from build123d import *

# Parameters (mm, degrees)
BOSS_EXTRUDE3_DEPTH = 6


with BuildPart() as part:
    # Sketch1 → Boss-Extrude3 (new body)
    with BuildSketch(Plane(origin=(0, 0, 0), x_dir=(1, 0, 0), z_dir=(0, 1, 0))):
        with BuildLine():
            ThreePointArc((-76.2, 131.982271537), (-131.982271537, 76.2), (-152.4, 0))
            Line((-152.4, 0), (-609.6, 0))
            ThreePointArc((-609.6, 0), (-527.929086147, 304.8), (-304.8, 527.929086147))
            Line((-304.8, 527.929086147), (-76.2, 131.982271537))
        make_face()
        with BuildLine():
            Line((-335.2, 10), (-599.516605275, 10))
            ThreePointArc((-599.516605275, 10), (-578.516992176, 157.601553812), (-521.750777563, 295.459449184))
            Line((-521.750777563, 295.459449184), (-335.2, 187.75430754))
            Line((-335.2, 187.75430754), (-335.2, 10))
        make_face(mode=Mode.SUBTRACT)
        with BuildLine():
            Line((-89.706166951, 135.375638912), (-171.260254038, 276.631461311))
            Line((-171.260254038, 276.631461311), (-325.2, 187.75430754))
            Line((-325.2, 187.75430754), (-325.2, 10))
            Line((-325.2, 10), (-162.091825827, 10))
            ThreePointArc((-162.091825827, 10), (-140.642525575, 81.2), (-89.706166951, 135.375638912))
        make_face(mode=Mode.SUBTRACT)
        with BuildLine():
            Line((-330.2, 196.414561578), (-516.750777563, 304.119703222))
            ThreePointArc((-516.750777563, 304.119703222), (-425.745445365, 422.209634839), (-308.418556675, 514.196610158))
            Line((-308.418556675, 514.196610158), (-176.260254038, 285.291715349))
            Line((-176.260254038, 285.291715349), (-330.2, 196.414561578))
        make_face(mode=Mode.SUBTRACT)
    extrude(amount=BOSS_EXTRUDE3_DEPTH)


solid = part.part
Could you check a few things on this model? Use its own coordinates, in mm. A direction names the side the tool comes from. Round coordinates to 2 decimals unless told otherwise and drop trailing zeros. Order: outer loops, then holes, each group sorted by start corner. A loop starts at its lowest first (then second) coordinate and runs counter-clockwise, first axis right, second up.
Q1. Imagine slicing it at A-A, the plane y = 3.6. List the corners of the cut face in (x, z) for me, then the cut area to 3 significant figures.
Geometry says:
outline: (-609.6, 0) arc R609.6 ccw to (-304.8, -527.93) - (-76.2, -131.98) arc R152.4 cw to (-152.4, 0) - close; hole (-599.52, -10) arc R599.6 ccw to (-521.75, -295.46) - (-335.2, -187.75) - (-335.2, -10) - close; hole (-516.75, -304.12) arc R599.6 ccw to (-308.42, -514.2) - (-176.26, -285.29) - (-330.2, -196.41) - close; hole (-325.2, -187.75) - (-171.26, -276.63) - (-89.71, -135.38) arc R162.4 cw to (-162.09, -10) - (-325.2, -10) - close
area: 22,500 mm2
Q2. Which directions (+Z, -Z, +X, -X, +Y, -Y) give clear straight access to the entire face, cutting with the end or side of a thin tool? Please do faces 4 (the face through (-427.22, 2.96, -420.72)), 5 (the face through (-361, 0, -207)).
Geometry says:
face 4: +Y, -Y
face 5: +Z, -Z, +X, -X, -Y
Q3. I'm going to push flat-ended pins straight in: P1, Ø1.8, axis at y = 2.5, z = -132, coming from the +X side; P2, Ø3, axis at x = -223, y = 1.5, coming from the -Z side; P3, Ø1.5, axis at x = -524.5, y = 5.5, coming from the -Z side; P4, Ø1.5, axis at x = -177.5, z = -285, coming from the -Y side. Where does each tip first touch, or does it pass through?
Geometry says:
P1: stops at x = -76.2
P2: stops at z = -388.85
P3: stops at z = -311.93
P4: stops at y = 0
Q4. Imagine slicing it at B-B, the plane x = -384. List the corners of the cut face in (y, z) for me, then the cut area to 3 significant figures.
Geometry says:
outline: (0, -473.45) - (6, -473.45) - (6, -460.5) - (0, -460.5) - close; (0, -227.48) - (6, -227.48) - (6, -215.93) - (0, -215.93) - close; (0, -10) - (6, -10) - (6, 0) - (0, 0) - close
area: 207 mm2
Q5. Imagine slicing it at C-C, the plane z = -230.5. List the corners of the cut face in (x, y) for me.
Geometry says:
outline: (-564.34, 0) - (-553.52, 0) - (-553.52, 6) - (-564.34, 6) - close; (-409.24, 0) - (-389.24, 0) - (-389.24, 6) - (-409.24, 6) - close; (-271.16, 0) - (-251.16, 0) - (-251.16, 6) - (-271.16, 6) - close; (-144.63, 0) - (-133.08, 0) - (-133.08, 6) - (-144.63, 6) - close
Q6. Imagine slicing it at D-D, the plane z = -433.5. List the corners of the cut face in (x, y) for me.
Geometry says:
outline: (-428.59, 0) - (-414.24, 0) - (-414.24, 6) - (-428.59, 6) - close; (-261.83, 0) - (-250.28, 0) - (-250.28, 6) - (-261.83, 6) - close
Q7. Thinking about a two-plate mould opening in X: for faces 1 (the face through (-247.153, 2.958, -232.815)), 2 (the face through (-131.4, 3, -77.2)), 3 (the face through (-361, 6, -207)), which applies, released by +X, released by -X, zero draft, split by the parting line, or undercut?
Geometry says:
face 1: undercut
face 2: released by +X
face 3: zero draft
Q8. Please list where these lines run through material, in increasing order: probe 1 along Z at (x, y) = (-471, 0.5); probe 2 along X at (y, z) = (1.9, -69.5); probe 3 along Z at (x, y) = (-463.5, 2.1).
Geometry says:
probe 1: z = -387 to -371.05, -277.71 to -266.16, -10 to 0
probe 2: x = -605.63 to -595.56, -335.2 to -325.2, -146.78 to -135.63
probe 3: z = -395.95 to -380.38, -273.38 to -261.83, -10 to 0
